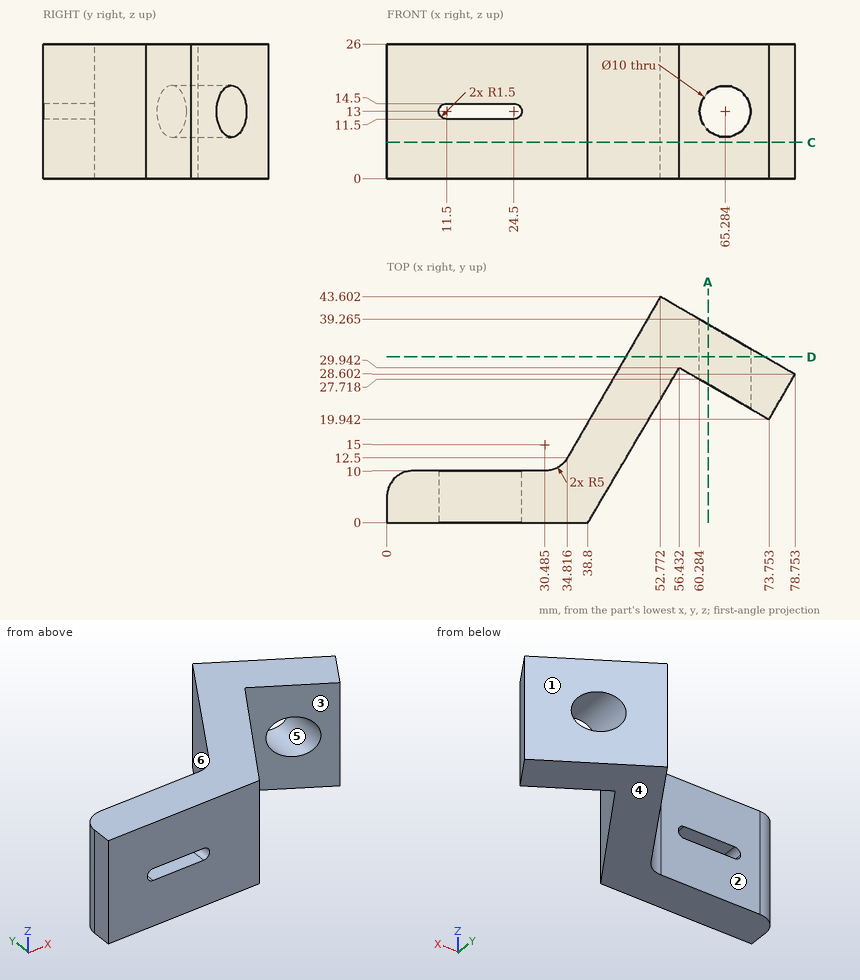
For this review, use the dimensioned drawing (mm, ordinates from the lowest corner) and the shaded views. A direction names the side the tool comes from. Give positions to 0.01 mm unless a question says otherwise; leave off trailing zeros. Order: outer loops, then holes, each group sorted by start corner. A loop starts at its lowest first (then second) coordinate and runs counter-clockwise, first axis right, second up. Notation, with made-up numbers: M 85.25,-9 L 138.25,-9 A24 cw 138.25,2 Z; hole C 40.5,62 d6. An arc over 180 degrees is marked long. One line per question, with ' | ' between items. Start each with the question number.
1) Consider section C-C, the plane z = 7. Give the boundary of the cut face in (x, y) (1 decimal), then the cut area to 3 significant figures.
2) Clearance check with flat-ended pins moving along their axes: P1, Ø1, axis at x = 59, z = 8, coming from the +Y side (1 decimal); P2, Ø7.5, axis at x = 18, z = 18.5, coming from the +Y side; P3, Ø3, axis at y = 23.5, z = 5, coming from the -X side. State where each tip first meets the part, or that it passes through.
3) Wall thickness on L1, parallel to X at y = 28, z = 13 (1 decimal); L2, parallel to Z at x = 14.5, y = 6.5; L3, parallel to X at y = 28.75, z = 13 (1 decimal): over which ranges is each line inside the solid? List them lowest first. Write a range as from..to.
4) Consider section A-A, the plane x = 62. Give the boundary of the cut face in (y, z) (1 decimal), then the cut area to 3 significant figures.
5) Consider section D-D, the plane y = 32. Give the boundary of the cut face in (x, z), then the cut area to 3 significant figures.
6) Mouldability with a two-part tool opening along X and no side actions: class the marked faces 4, 5 and 6 as pulls with the +X half, pulls with the -X half, needs draft (parallel to the pull), parting line crosses it, or undercut.
7) For the marked faces 1, 2 and 3, list the 3-axis set-ups (+Z, -Z, +X, -X, +Y, -Y) from which the entire face can be reached by the end or side of a thin tool; tool diameter is ignored.
Found:
1) outline: M 0,0 L 38.8,0 L 56.4,29.9 L 73.8,19.9 L 78.8,28.6 L 52.8,43.6 L 34.8,12.5 A5 cw 30.5,10 L 5,10 A5 ccw 0,5 Z | area: 970 mm²
2) P1: stops at y = 40.3 | P2: stops at y = 10 | P3: stops at x = 40.3
3) L1: x = 43.8..55.3, 59.8..60.3, 70.3..78.4 | L2: z = 0..11.5, 14.5..26 | L3: x = 44.2..55.7, 58.5..60.3, 70.3..78.5
4) outline: M 26.7,0 L 38.3,0 L 38.3,9.2 L 26.7,9.2 Z; M 26.7,16.8 L 38.3,16.8 L 38.3,26 L 26.7,26 Z | area: 213 mm²
5) outline: M 46.07,0 L 72.87,0 L 72.87,26 L 46.07,26 Z; hole C 65.28,13 d10 | area: 618 mm²
6) face 4: needs draft | face 5: undercut | face 6: pulls with the -X half
7) face 1: +Z, -Z, +X, +Y | face 2: +Z, -Z, -X, +Y | face 3: +Z, -Z, -Y
